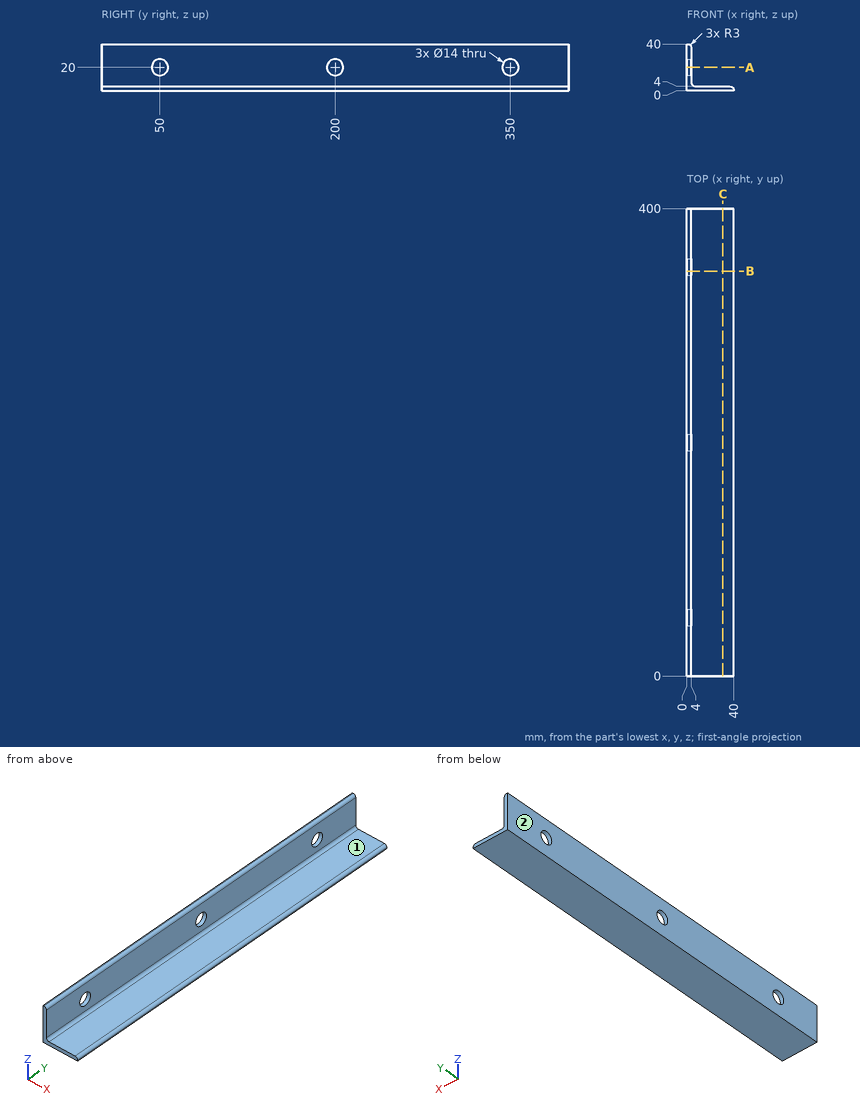
Here's the drawing with two shaded views (mm, measured from the low corner). I have some questions. A direction names the side the tool comes from. Coordinates: 2 decimals unless noted, no trailing zeros. Loops run counter-clockwise (first coordinate to the right, second up) from the corner with the lowest first, then second, coordinate; pieces in that order, holes last.
Item 1: Which directions (+Z, -Z, +X, -X, +Y, -Y) give clear straight access to the entire face, cutting with the end or side of a thin tool? Please do the marked faces 1 and 2.
Answers below:
face 1: +Z, +X, +Y, -Y
face 2: +Z, -Z, -X, +Y, -Y
Item 2: Please list where these lines run through material, in increasing order: L1, parallel to Y at x = 2, z = 20; L2, parallel to X at y = 36, z = 12.5.
Answers below:
L1: y = 0 to 43, 57 to 193, 207 to 343, 357 to 400
L2: x = 0 to 4
Item 3: Suppose I cut it at B-B (y = 346.5). Please give me the cut outline in (x, z).
Answers below:
outline: (0, 0) - (40, 0) - (40, 1) arc R3 ccw to (37, 4) - (7, 4) arc R3 cw to (4, 7) - (4, 13.94) - (0, 13.94) - close; (0, 26.06) - (4, 26.06) - (4, 37) arc R3 ccw to (1, 40) - (0, 40) - close
Item 4: Suppose I cut it at C-C (x = 31). Please give me the cut outline in (y, z), then the cut area to 3 significant figures.
Answers below:
outline: (0, 0) - (400, 0) - (400, 4) - (0, 4) - close
area: 1,600 mm2
Item 5: I'm going to push flat-ended pins straight in: pin 1 (3 mm diameter, centred on y = 351.5, z = 8.5, fed in from +X); pin 2 (3 mm diameter, centred on x = 31, y = 214.5, fed in from +Z); pin 3 (5 mm diameter, centred on y = 58.5, z = 5.5, fed in from +X); pin 4 (12.5 mm diameter, centred on y = 350, z = 20, fed in from +X). Where does each tip first touch, or does it pass through?
Answers below:
pin 1: stops at x = 4
pin 2: stops at z = 4
pin 3: stops at x = 39.24
pin 4: passes through
Item 6: Suppose I cut it at A-A (z = 20). Please give me the cut outline in (x, y).
Answers below:
outline: (0, 0) - (4, 0) - (4, 43) - (0, 43) - close; (0, 57) - (4, 57) - (4, 193) - (0, 193) - close; (0, 207) - (4, 207) - (4, 343) - (0, 343) - close; (0, 357) - (4, 357) - (4, 400) - (0, 400) - close
